```python
from build123d import *

# Parameters (mm, degrees)
SKETCH1_R           = 4.025
SKETCH1_R_2         = 0.75
SKETCH1_W           = 5
SKETCH1_H           = 10
BOSS_EXTRUDE1_DEPTH = 5
CUT_EXTRUDE1_DEPTH  = 10
CUT_EXTRUDE2_DEPTH  = 10


with BuildPart() as part:
    # Sketch1 → Boss-Extrude1 (new body)
    with BuildSketch(Plane.XY):
        with BuildLine():
            Line((-215, 15), (-60, 15))
            ThreePointArc((-60, 15), (-56.464466094, 13.535533906), (-55, 10))
            Line((-55, 10), (-55, 5))
            ThreePointArc((-55, 5), (-56.464466094, 1.464466094), (-60, 0))
            Line((-60, 0), (-215, 0))
            ThreePointArc((-215, 0), (-218.535533906, 1.464466094), (-220, 5))
            Line((-220, 5), (-220, 10))
            ThreePointArc((-220, 10), (-218.535533906, 13.535533906), (-215, 15))
        make_face()
        with Locations((-212.5, 7.5)):
            Circle(SKETCH1_R, mode=Mode.SUBTRACT)
        with Locations((-204.75, 7.5)):
            Circle(SKETCH1_R_2, mode=Mode.SUBTRACT)
        with Locations((-201.75, 7.5)):
            Circle(SKETCH1_R_2, mode=Mode.SUBTRACT)
        with Locations((-198.75, 7.5)):
            Circle(SKETCH1_R_2, mode=Mode.SUBTRACT)
        with Locations((-62.5, 7.5)):
            Rectangle(SKETCH1_W, SKETCH1_H, mode=Mode.SUBTRACT)
    extrude(amount=BOSS_EXTRUDE1_DEPTH)

    # Sketch2 → Cut-Extrude1 (cut)
    with BuildSketch(Plane(origin=(0, 0, 0), x_dir=(-1, 0, 0), z_dir=(0, 0, -1))):
        Polygon((65, 9.6), (71.8, 9.6), (71.8, 11), (75, 11), (75, 9.6), (82, 9.6), (82, 5.4), (75, 5.4), (75, 4), (71.8, 4), (71.8, 5.4), (65, 5.4), align=None)
    extrude(amount=-CUT_EXTRUDE1_DEPTH, mode=Mode.SUBTRACT)

    # Sketch3 → Cut-Extrude2 (cut)
    with BuildSketch(Plane(origin=(0, 0, 0), x_dir=(-1, 0, 0), z_dir=(0, 0, -1))):
        with BuildLine():
            Line((60, 15), (60, 0))
            ThreePointArc((60, 0), (56.464466094, 1.464466094), (55, 5))
            Line((55, 5), (55, 10))
            ThreePointArc((55, 10), (56.464466094, 13.535533906), (60, 15))
        make_face()
    extrude(amount=-CUT_EXTRUDE2_DEPTH, mode=Mode.SUBTRACT)


solid = part.part
```
Work out the finished part from the listing and answer in its coordinate system (mm). A direction names the side the tool comes from. Round coordinates to 2 decimals unless told otherwise and drop trailing zeros. Write each loop counter-clockwise with the first axis right and the second up, starting at its lowest first coordinate (ties: lowest second). Pieces come first, ordered by that corner, then holes.
1) A cutting plane is placed at A-A on x = -80. Determine the outline of the cut face in (y, z), and give its area (3 significant figures).
2) Flat-ended cylindrical pins translate along their axes: P1, Ø0.7, axis at y = 10.5, z = 3, coming from the -X side; P2, Ø3, axis at y = 4.5, z = 3, coming from the +X side; P3, Ø2, axis at y = 8.5, z = 1, coming from the +X side; P4, Ø4, axis at x = -177.5, y = 5.5, coming from the -Z side. Find the tip coordinate at first contact, or state that the pin passes through.
3) Consider probe 1 along X at (y, z) = (5, 1.2); probe 2 along Y at (x, z) = (-212.5, 1.25) (3 decimals); probe 3 along X at (y, z) = (10.25, 0.7). Determine where each line is inside the solid, lowest interval first.
4) Which of the six approach directions +Z, -Z, +X, -X, +Y, -Y give full straight-line access (tool end or side, diameter ignored) to faces 4 (the face through (-73, 4, 2)), 5 (the face through (-60, 1, 2)), 6 (the face through (-65, 4, 2))?
5) A cutting plane is placed at C-C on x = -212.5. Determine the outline of the cut face in (y, z) (3 decimals).
6) Determine the mould class of faces 1 (the face through (-139, 8, 5)), 2 (the face through (-82, 8, 2)), 3 (the face through (-139, 15, 2)) for opening direction Y: pulls with the +Y half, pulls with the -Y half, needs draft (parallel to the pull), parting line crosses it, or undercut.
7) A cutting plane is placed at B-B on z = 1.5. Determine the outline of the cut face in (x, y) (3 decimals).
Entries:
1. outline: (0, 0) - (5.4, 0) - (5.4, 5) - (0, 5) - close; (9.6, 0) - (15, 0) - (15, 5) - (9.6, 5) - close
1. area: 54.0 mm2
2. P1: stops at x = -220
2. P2: stops at x = -65
2. P3: stops at x = -82
2. P4: stops at z = 0
3. probe 1: x = -220 to -215.65, -209.35 to -75, -71.8 to -65
3. probe 2: y = 0 to 3.475, 11.525 to 15
3. probe 3: x = -219.99 to -215.44, -209.56 to -75, -71.8 to -65
4. face 4: +Z, -Z
4. face 5: +Z, -Z, +X, +Y, -Y
4. face 6: +Z, -Z, +X
5. outline: (0, 0) - (3.475, 0) - (3.475, 5) - (0, 5) - close; (11.525, 0) - (15, 0) - (15, 5) - (11.525, 5) - close
6. face 1: needs draft
6. face 2: undercut
6. face 3: pulls with the +Y half
7. outline: (-220, 5) arc R5 ccw to (-215, 0) - (-60, 0) - (-60, 2.5) - (-65, 2.5) - (-65, 5.4) - (-71.8, 5.4) - (-71.8, 4) - (-75, 4) - (-75, 5.4) - (-82, 5.4) - (-82, 9.6) - (-75, 9.6) - (-75, 11) - (-71.8, 11) - (-71.8, 9.6) - (-65, 9.6) - (-65, 12.5) - (-60, 12.5) - (-60, 15) - (-215, 15) arc R5 ccw to (-220, 10) - close; hole circle Ø8.05 at (-212.5, 7.5); hole circle Ø1.5 at (-204.75, 7.5); hole circle Ø1.5 at (-201.75, 7.5); hole circle Ø1.5 at (-198.75, 7.5)
